Source: CAD feature listing. Evaluate the final solid. Frame: model axes, mm. A direction names the side the tool comes from. Round coordinates to 2 decimals unless told otherwise and drop trailing zeros. Order: outer loops, then holes, each group sorted by start corner. A loop starts at its lowest first (then second) coordinate and runs counter-clockwise, first axis right, second up. Notation, with made-up numbers: (-12, 31) - (3, 31) arc R18 ccw to (3, 45) - close; hole circle Ø3 at (43, 42.5). An arc over 180 degrees is marked (long way). Put each result on its own line as item: value. Start each with the question number.
1) Line query: probe 1 along Z at (x, y) = (36, 4); probe 2 along Y at (x, z) = (50, -18). Output: solid intervals per line, ascending. Write a range as [from, to].
2) Section B-B on x = 35.5. Output: boundary loops of the cut face in (y, z).
3) Mould query, pull axis X, two halves, no side actions, for faces 1 (the face through (36.1, 4.97, -22.82)), 2 (the face through (27, 46.5, -20)), 3 (the face through (0.57, 23.58, -0.6)). Classes: +X half, -X half, draft (parallel to the pull), parting line (faces both ways), or undercut.
4) Section A-A on y = 3. Output: boundary loops of the cut face in (x, z), then the cut area to 3 significant figures.
5) Contact query for a flat-ended pin moving along its axis: P1, Ø4, axis at x = 22.5, z = -19, coming from the -Y side. Output: stop coordinate, or through.
6) Section C-C on z = -27. Output: boundary loops of the cut face in (x, y).
7) Access query for faces 4 (the face through (36.568, 4.974, -16.825)), 5 (the face through (0.57, 23.58, -38.65)). Directions: +Z, -Z, +X, -X, +Y, -Y. A direction counts if a zero-diameter tool reaches every point of the face in a straight line with its end or side. Return the directions, or none.
```python
from build123d import *

# Parameters (mm, degrees)
SKETCH1_W              = 54
SKETCH1_H              = 39.25
BOSS_EXTRUDE1_DEPTH    = 46.5
FILLET1_R              = 2
FILLET2_R              = 2
Z_95_START             = -0.023652431
Z_95_BLANK_DEPTH       = 10
Z_95_START_2           = -5.023652431
Z_95_BLANK_2_OUTLINE_R = 2.5
Z_95_BLANK_2_DEPTH     = 5
BODY_MOVE_COPY3_ANGLE  = 180
BODY_MOVE_COPY4_ANGLE  = 89.5


with BuildPart() as part:
    # Sketch1 → Boss-Extrude1 (new body)
    with BuildSketch(Plane(origin=(0, 0, 0), x_dir=(1, 0, 0), z_dir=(0, 1, 0))):
        with Locations((27, 19.625)):
            Rectangle(SKETCH1_W, SKETCH1_H)
    extrude(amount=BOSS_EXTRUDE1_DEPTH)

    # Fillet1
    fillet1_edges = [part.edges().sort_by_distance(p)[0] for p in [
        (0, 23.25, 0),
    ]]
    fillet(fillet1_edges, radius=FILLET1_R)

    # Fillet2
    fillet2_edges = [part.edges().sort_by_distance(p)[0] for p in [
        (0, 23.25, -39.25),
        (54, 23.25, -39.25),
        (54, 23.25, 0),
    ]]
    fillet(fillet2_edges, radius=FILLET2_R)


with BuildPart() as body_2:
    # Z-95 Blank: read off the stored shape, not the designer's step
    # Z-95 Blank outline → Z-95 Blank (new body)
    with BuildSketch(Plane(origin=(0, 0, 0), x_dir=(1, 0, 0), z_dir=(0, 1, 0)).offset(Z_95_START)):
        Polygon((-39.475833264, 51.689675598), (-39.475833264, 48.062948495), (-51.475833264, 46.678320586), (-51.475833264, 23.139646129), (-47.225833264, 23.139646129), (-47.225833264, 35.139646129), (-37.225833264, 35.139646129), (-35.725833264, 5.689675598), (-31.225833264, 5.689675598), (-29.725833264, 35.139646129), (-19.725833264, 35.139646129), (-19.725833264, 23.139646129), (-15.475833264, 23.139646129), (-15.475833264, 46.678320586), (-27.475833264, 48.062948495), (-27.475833264, 51.689675598), align=None)
    extrude(amount=Z_95_BLANK_DEPTH)

    # Z-95 Blank 2 outline → Z-95 Blank 2 (add)
    with BuildSketch(Plane(origin=(0, 0, 0), x_dir=(1, 0, 0), z_dir=(0, 1, 0)).offset(Z_95_START_2)):
        with Locations((-33.475833264, 34.343753809)):
            Circle(Z_95_BLANK_2_OUTLINE_R)
    extrude(amount=Z_95_BLANK_2_DEPTH)


with BuildPart() as body_2_1:
    # Body-Move/Copy3: moved
    add(body_2.part.rotate(Axis((0, 2.476347569, -28.689675598), (1, 0, 0)), BODY_MOVE_COPY3_ANGLE))


with BuildPart() as body_2_2:
    # Body-Move/Copy4: moved
    add(body_2_1.part.rotate(Axis((-33.475833264, 0, -28.689675598), (0, -1, 0)), BODY_MOVE_COPY4_ANGLE))


with BuildPart() as body_2_3:
    # Body-Move/Copy5: moved
    add(body_2_2.part.moved(Location((61.536777905, 5.06338101, 8.948981511))))


with BuildPart() as body_2_4:
    # Body-Move/Copy6: moved
    add(body_2_3.part.moved(Location((0, -0.229742035, 0))))


with BuildPart() as part_1:
    add(part.part)

    # Intersect1: read off the stored shape, not the designer's step
    # Intersect1: cut body 2
    add(body_2_4.part, mode=Mode.SUBTRACT)


solid = part_1.part
```
Answer sheet:
1. probe 1: [-39.25, -22.83], [-16.79, 0]
1. probe 2: [9.81, 46.5]
2. outline: (0, -39.25) - (46.5, -39.25) - (46.5, 0) - (0, 0) - (0, -16.76) - (9.81, -16.76) - (9.81, -22.85) - (0, -22.85) - close
3. face 1: undercut
3. face 2: draft
3. face 3: -X half
4. outline: (0, -37.25) arc R2 ccw to (2, -39.25) - (52, -39.25) arc R2 ccw to (54, -37.25) - (54, -2) arc R2 ccw to (52, 0) - (2, 0) arc R2 ccw to (0, -2) - close; hole (5.01, -25.54) - (8.64, -25.57) - (9.92, -37.58) - (33.45, -37.79) - (33.49, -33.54) - (21.49, -33.43) - (21.58, -23.43) - (51.04, -22.19) - (51.08, -17.69) - (21.64, -15.93) - (21.73, -5.93) - (33.73, -6.04) - (33.77, -1.79) - (10.23, -1.58) - (8.74, -13.57) - (5.11, -13.54) - close
4. area: 1,350 mm^2
5. P1: y = 9.81
6. outline: (0, 0) - (8.79, 0) - (8.79, 9.81) - (21.55, 9.81) - (21.55, 0) - (54, 0) - (54, 46.5) - (0, 46.5) - close
7. face 4: -Y
7. face 5: -Z, -X, +Y, -Y
